Design review of the part built by this model. Coordinates are the model's own, in mm. Give positions to 0.01 mm unless a question says otherwise; leave off trailing zeros. Loops run counter-clockwise (first coordinate to the right, second up) from the corner with the lowest first, then second, coordinate; pieces in that order, holes last.
from build123d import *

# Parameters (mm, degrees)
SKETCH_2_W      = 45
SKETCH_2_H      = 160
EXTRUDE_1_DEPTH = 3


with BuildPart() as part:
    # Эскиз2 → Бобышка-Вытянуть1 (new, symmetric)
    with BuildSketch(Plane(origin=(0, 0, 0), x_dir=(1, 0, 0), z_dir=(0, 1, 0))):
        Rectangle(SKETCH_2_W, SKETCH_2_H)
        with BuildLine():
            Line((-5, 63), (-5, 71))
            ThreePointArc((-5, 71), (0, 76), (5, 71))
            Line((5, 71), (5, 63))
            ThreePointArc((5, 63), (0, 58), (-5, 63))
        make_face(mode=Mode.SUBTRACT)
        with BuildLine():
            Line((-5, -63), (-5, -71))
            ThreePointArc((-5, -71), (0, -76), (5, -71))
            Line((5, -71), (5, -63))
            ThreePointArc((5, -63), (0, -58), (-5, -63))
        make_face(mode=Mode.SUBTRACT)
    extrude(amount=EXTRUDE_1_DEPTH, both=True)


solid = part.part
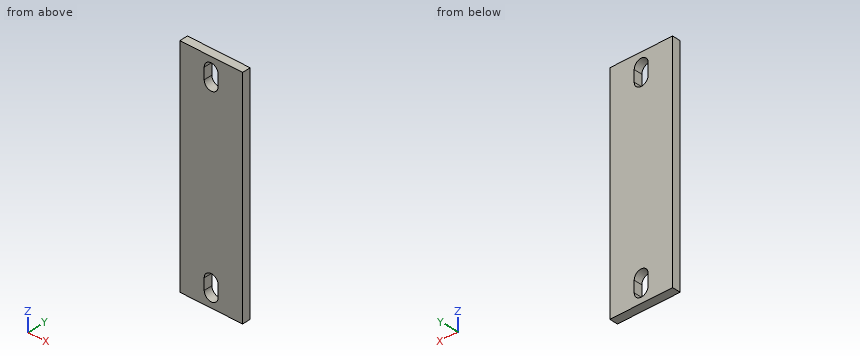
Q1. Take a section at B-B (y = 1.35). Give the boundary of the cut face in (x, z), plus the area to 3 significant figures.
Results:
outline: (-22.5, -80) - (22.5, -80) - (22.5, 80) - (-22.5, 80) - close; hole (-5, -71) arc R5 ccw to (5, -71) - (5, -63) arc R5 ccw to (-5, -63) - close; hole (-5, 63) arc R5 ccw to (5, 63) - (5, 71) arc R5 ccw to (-5, 71) - close
area: 6,880 mm2
Q2. Wall thickness on line 1 (X direction, y = -1.3, z = 64); line 2 (Z direction, x = -0.5, y = -0.7); line 3 (Z direction, x = -3.5, y = 1.3): over which ranges is each line inside the solid? List them lowest first.
Results:
line 1: x = -22.5 to -5, 5 to 22.5
line 2: z = -80 to -75.97, -58.03 to 58.03, 75.97 to 80
line 3: z = -80 to -74.57, -59.43 to 59.43, 74.57 to 80
Q3. Take a section at A-A (x = 0). Give the boundary of the cut face in (y, z), plus the area to 3 significant figures.
Results:
outline: (-3, -80) - (3, -80) - (3, -76) - (-3, -76) - close; (-3, -58) - (3, -58) - (3, 58) - (-3, 58) - close; (-3, 76) - (3, 76) - (3, 80) - (-3, 80) - close
area: 744 mm2
